Verification items for the finished model (mm, model axes). A direction names the side the tool comes from. Round coordinates to 2 decimals unless told otherwise and drop trailing zeros. Order: outer loops, then holes, each group sorted by start corner. A loop starts at its lowest first (then second) coordinate and runs counter-clockwise, first axis right, second up. Notation, with made-up numbers: (3.5, 58) -> (49.5, 58) arc R18 cw to (49.5, 86) -> close; hole circle Ø4 at (39, 57.5). An arc over 180 degrees is marked (long way). Put each result on its own line as item: value.
from build123d import *

# Parameters (mm, degrees)
SKETCH1_R           = 1.5
BOSS_EXTRUDE1_DEPTH = 17.1
SKETCH2_R           = 2.25
BOSS_EXTRUDE2_DEPTH = 3
BOSS_EXTRUDE3_START = -17.1
SKETCH2_2_R         = 2.25
BOSS_EXTRUDE3_DEPTH = 3


with BuildPart() as part:
    # Sketch1 → Boss-Extrude1 (new body)
    with BuildSketch(Plane(origin=(0, 0, 0), x_dir=(1, 0, 0), z_dir=(0, 1, 0))):
        Circle(SKETCH1_R)
    extrude(amount=BOSS_EXTRUDE1_DEPTH)

    # Sketch2 → Boss-Extrude2 (add)
    with BuildSketch(Plane(origin=(0, 17.1, 0), x_dir=(1, 0, 0), z_dir=(0, 1, 0))):
        Circle(SKETCH2_R)
    extrude(amount=BOSS_EXTRUDE2_DEPTH)

    # Sketch2<2> → Boss-Extrude3 (add)
    with BuildSketch(Plane(origin=(0, 17.1, 0), x_dir=(1, 0, 0), z_dir=(0, 1, 0)).offset(BOSS_EXTRUDE3_START)):
        Circle(SKETCH2_2_R)
    extrude(amount=-BOSS_EXTRUDE3_DEPTH)


solid = part.part
Item 1: Section check A-A on x = 0. Record the boundary of the cut face in (y, z), then the cut area to 3 significant figures.
Check sheet entries:
outline: (-3, -2.25) -> (0, -2.25) -> (0, -1.5) -> (17.1, -1.5) -> (17.1, -2.25) -> (20.1, -2.25) -> (20.1, 2.25) -> (17.1, 2.25) -> (17.1, 1.5) -> (0, 1.5) -> (0, 2.25) -> (-3, 2.25) -> close
area: 78.3 mm^2
Item 2: Gauge pin test, flat ends, axial feed: pin 1 Ø1.5 at (x, y) = (0, 15.5) entering from -Z; pin 2 Ø1.5 at (y, z) = (7.5, -1.5) entering from -X; pin 3 Ø1 at (y, z) = (6, 1.5) entering from +X. Record the tip position at first contact, or that the pin passes through.
Check sheet entries:
pin 1: stops at z = -1.5
pin 2: stops at x = -1.3
pin 3: stops at x = 1.12
Item 3: Release check for a two-part mould opening along Y. For faces 3 (the flat face through (0, 20.1, 0)), 4 (the flat face through (0, -3, 0)), 5 (the cylindrical face through (-0.29, -1.48, -2.23)), 6 (the cylindrical face through (-1.5, 8.43, -0.07)) record: +Y half, -Y half, draft (parallel to the pull), parting line (faces both ways), or undercut.
Check sheet entries:
face 3: +Y half
face 4: -Y half
face 5: draft
face 6: undercut
Item 4: Tool access check on faces 1 (the cylindrical face through (-0.29, 18.58, -2.23)), 2 (the flat face through (-2, 0, 0)). Record the directions out of +Z, -Z, +X, -X, +Y, -Y that give a thin tool (end or side, any length) a straight path to the whole face; none if there is none.
Check sheet entries:
face 1: +Y, -Y
face 2: none
Item 5: Section check B-B on z = 0. Record the boundary of the cut face in (x, y).
Check sheet entries:
outline: (-2.25, -3) -> (2.25, -3) -> (2.25, 0) -> (1.5, 0) -> (1.5, 17.1) -> (2.25, 17.1) -> (2.25, 20.1) -> (-2.25, 20.1) -> (-2.25, 17.1) -> (-1.5, 17.1) -> (-1.5, 0) -> (-2.25, 0) -> close
Item 6: Material ranges on L1, parallel to Y at x = -1.35, z = -1.1; L2, parallel to X at y = 3.5, z = 0.05; L3, parallel to X at y = 3, z = 1.35, recorded low to high. Write a range as [from, to].
Check sheet entries:
L1: y = [-3, 0], [17.1, 20.1]
L2: x = [-1.5, 1.5]
L3: x = [-0.65, 0.65]
Item 7: Section check C-C on y = 11. Record the boundary of the cut face in (x, z), then the cut area to 3 significant figures.
Check sheet entries:
outline: circle Ø3 at (0, 0)
area: 7.07 mm^2
